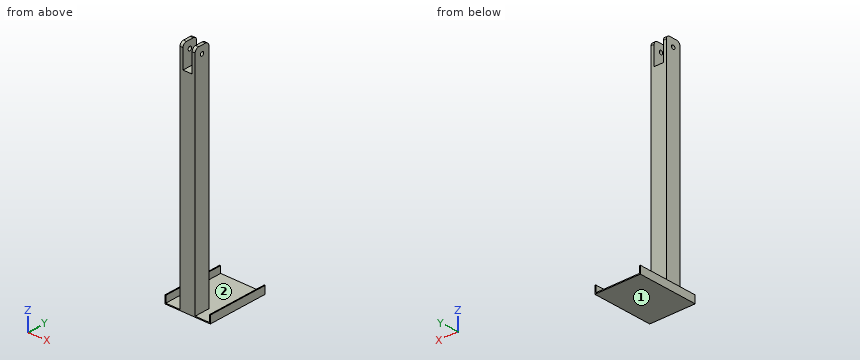
```python
from build123d import *

# Parameters (mm, degrees)
F1_DEPTH = 101.6
F2_W     = 50.8
F2_H     = 50.8
F3_DEPTH = 762
F4_R     = 6.35
F5_DEPTH = 101.601
F6_W     = 30.48
F6_H     = 76.2
F7_DEPTH = 203.201
F8_R     = 12.7


with BuildPart() as f1:
    # F0 (on Front) → F1 (new body, symmetric)
    with BuildSketch(Plane.XZ):
        Polygon((-73.025, 25.4), (-76.2, 25.4), (-76.2, 0), (76.2, 0), (76.2, 25.4), (73.025, 25.4), (73.025, 3.175), (-73.025, 3.175), align=None)
    extrude(amount=F1_DEPTH, both=True)

    # F2 (on face) → F3 (join)
    with BuildSketch(Plane.XY.offset(3.175)):
        with Locations((0, -76.2)):
            Rectangle(F2_W, F2_H)
    extrude(amount=F3_DEPTH)

    # F4 (on face) → F5 (cut, through all)
    with BuildSketch(Plane.YZ.offset(25.4)):
        with Locations((-76.2, 739.775)):
            Circle(F4_R)
    extrude(amount=-F5_DEPTH, mode=Mode.SUBTRACT)

    # F6 (on face) → F7 (cut, through all)
    with BuildSketch(Plane.XZ.offset(101.6)):
        with Locations((0, 727.075)):
            Rectangle(F6_W, F6_H)
    extrude(amount=-F7_DEPTH, mode=Mode.SUBTRACT)

    # F8
    f8_edges = [f1.edges().sort_by_distance(p)[0] for p in [
        (-20.32, -101.6, 765.175),
        (20.32, -101.6, 765.175),
        (-20.32, -50.8, 765.175),
        (20.32, -50.8, 765.175),
    ]]
    fillet(f8_edges, radius=F8_R)


solid = f1.part
```
Design review of the part built by this model. Coordinates are the model's own, in mm. Face numbers are marked on the shaded views. Round coordinates to 2 decimals unless told otherwise and drop trailing zeros. Order: outer loops, then holes, each group sorted by start corner. A loop starts at its lowest first (then second) coordinate and runs counter-clockwise, first axis right, second up. Notation, with made-up numbers: (82.5, -35) - (117.5, -35) arc R11 cw to (117.5, -27) - close; hole circle Ø5 at (-21.5, -31.5). An arc over 180 degrees is marked (long way). Return JSON: item names as keys, results as strings.
Q1. Consider section B-B on x = 40. Write out the cut boundary in (y, z) (3 decimals), plus the area to 3 significant figures.
Computed values:
{"outline": "(-101.6, 0) - (101.6, 0) - (101.6, 3.175) - (-101.6, 3.175) - close", "area": "645 mm2"}
Q2. The part is to be moulded in two halves that separate along X. For the marked faces 1 and 2, say which applies: pulls with the +X half, pulls with the -X half, needs draft (parallel to the pull), parting line crosses it, or undercut.
Computed values:
{"face 1": "needs draft", "face 2": "undercut"}
Q3. Consider section C-C on z = 81. Write out the cut boundary in (x, y).
Computed values:
{"outline": "(-25.4, -101.6) - (25.4, -101.6) - (25.4, -50.8) - (-25.4, -50.8) - close"}
Q4. Wall thickness on L1, parallel to Z at x = 22.5, y = -76 (3 decimals); L2, parallel to Z at x = 28, y = 73.5 (3 decimals); L3, parallel to Y at x = 5.5, z = 273.5: over which ranges is each line inside the solid? List them lowest first. Write a range as [from, to].
Computed values:
{"L1": "z = [0, 733.428], [746.122, 765.175]", "L2": "z = [0, 3.175]", "L3": "y = [-101.6, -50.8]"}
Q5. For pin 1 Ø2.5 at (x, y) = (-74, -27) entering from +Z; pin 2 Ø3 at (x, z) = (20, 562.5) entering from +Y; pin 3 Ø15 at (y, z) = (-77.5, 491) entering from +X, all flat-tipped, find the tip position at first contact; note any pin that passes through.
Computed values:
{"pin 1": "stops at z = 25.4", "pin 2": "stops at y = -50.8", "pin 3": "stops at x = 25.4"}
Q6. Consider section A-A on y = -10.5. Write out the cut boundary in (x, z) (3 decimals), plus the area to 3 significant figures.
Computed values:
{"outline": "(-76.2, 0) - (76.2, 0) - (76.2, 25.4) - (73.025, 25.4) - (73.025, 3.175) - (-73.025, 3.175) - (-73.025, 25.4) - (-76.2, 25.4) - close", "area": "625 mm2"}
